from build123d import *

# Parameters (mm, degrees)
SKETCH061_R     = 2.3
PAD042_DEPTH    = 3
PAD043_DEPTH    = 1.5
POCKET012_DEPTH = 0.6
CHAMFER006_SIZE = 0.1


with BuildPart() as part:
    # Sketch061 → Pad042 (new body)
    with BuildSketch(Plane.XY):
        Circle(SKETCH061_R)
    extrude(amount=PAD042_DEPTH)

    # Sketch062 (on Face3 of Pad042) → Pad043 (join)
    with BuildSketch(Plane.XY.offset(3)):
        with BuildLine():
            Line((0.425, 2.767558), (0.425, 3.617558))
            Line((0.425, 3.617558), (-0.425, 3.617558))
            Line((-0.425, 3.617558), (-0.425, 2.767558))
            ThreePointArc((-0.425, 2.767558), (0, -2.8), (0.425, 2.767558))
        make_face()
    extrude(amount=PAD043_DEPTH)

    # Sketch063 → Pocket012 (cut)
    with BuildSketch(Plane.XY):
        Polygon((-0.5, 0.5), (-1.5, 0.5), (-1.5, -0.5), (-0.5, -0.5), (-0.5, -1.5), (0.5, -1.5), (0.5, -0.5), (1.5, -0.5), (1.5, 0.5), (0.5, 0.5), (0.5, 1.5), (-0.5, 1.5), align=None)
    extrude(amount=POCKET012_DEPTH, mode=Mode.SUBTRACT)

    # Chamfer006
    chamfer006_edges = [part.edges().sort_by_distance(p)[0] for p in [
        (-1, 0.5, 0),
        (-2.3, 0, 0),
        (-1.5, 0, 0),
        (-1, -0.5, 0),
        (-0.5, -1, 0),
        (0, -1.5, 0),
        (0.5, -1, 0),
        (1, -0.5, 0),
        (1.5, 0, 0),
        (1, 0.5, 0),
        (0.5, 1, 0),
        (0, 1.5, 0),
        (-0.5, 1, 0),
    ]]
    chamfer(chamfer006_edges, length=CHAMFER006_SIZE)


with BuildPart() as part_1:
    # Body018 placement: moved
    add(part.part.moved(Location((63.6, 11.5, -1.5))))


solid = part_1.part
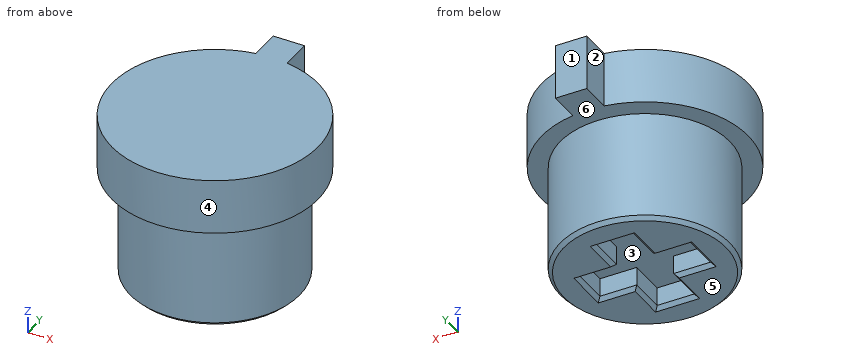
Work out the finished part from the listing and answer in its coordinate system (mm). Face numbers are marked on the shaded views. A direction names the side the tool comes from. Round coordinates to 2 decimals unless told otherwise and drop trailing zeros. Loops run counter-clockwise (first coordinate to the right, second up) from the corner with the lowest first, then second, coordinate; pieces in that order, holes last. Notation, with made-up numbers: (7, 80) - (59, 80) arc R22 cw to (59, 102) - close; hole circle Ø10 at (74.5, 6). An arc over 180 degrees is marked (long way). Use one line per item in the form item = value. Start each with the question number.
(1) Flat-ended cylindrical pins translate along their axes: P1, Ø0.5, axis at x = 62.5, z = -1, coming from the -Y side; P2, Ø0.5, axis at y = 12.5, z = -1, coming from the +X side; P3, Ø0.5, axis at x = 63.5, z = -1.5, coming from the +Y side. Find the tip coordinate at first contact, or state that the pin passes through.
(2) Find section C-C on y = 14.75. Determine the outline of the cut face in (x, z) (3 decimals), and give its area (4 significant figures).
(3) Find section B-B on z = 0.6. Determine the outline of the cut face in (x, y).
(4) Consider line 1 (Z direction, x = 65.8, y = 13); line 2 (Z direction, x = 64.1, y = 11.5); line 3 (X direction, y = 14.5, z = 2.3) (3 decimals). Determine where each line is inside the solid, lowest interval first.
(5) Determine the mould class of the marked faces 1, 2, 3 and 4 for opening direction X: +X half, -X half, draft (parallel to the pull), parting line (faces both ways), or undercut.
(6) Which of the six approach directions +Z, -Z, +X, -X, +Y, -Y give full straight-line access (tool end or side, diameter ignored) to the marked faces 5 and 6?
(7) Find section D-D on z = 2.25. Determine the outline of the cut face in (x, y) (3 decimals).
(8) Find section A-A on x = 63.6. Determine the outline of the cut face in (y, z).
Answer list:
q1.P1 = 9.36
q1.P2 = 65.77
q1.P3 = 13.8
q2.outline = (63.175, 1.5) - (64.025, 1.5) - (64.025, 3) - (63.175, 3) - close
q2.area = 1.275 mm^2
q3.outline = circle Ø4.6 at (63.6, 11.5)
q4.line_1 = 1.5 to 3
q4.line_2 = -0.9 to 3
q4.line_3 = 63.175 to 64.025
q5.face_1 = draft
q5.face_2 = -X half
q5.face_3 = undercut
q5.face_4 = parting line
q6.face_5 = -Z, +X, -X, +Y, -Y
q6.face_6 = -Z
q7.outline = (63.175, 14.268) arc R2.8 ccw (long way) to (64.025, 14.268) - (64.025, 15.118) - (63.175, 15.118) - close
q8.outline = (8.7, 1.5) - (9.2, 1.5) - (9.2, -1.4) - (9.3, -1.5) - (9.9, -1.5) - (10, -1.4) - (10, -0.9) - (13, -0.9) - (13, -1.4) - (13.1, -1.5) - (13.7, -1.5) - (13.8, -1.4) - (13.8, 1.5) - (15.12, 1.5) - (15.12, 3) - (8.7, 3) - close
